Geometry: final body of the model. Coordinates: model frame, mm. A direction names the side the tool comes from. Give positions to 0.01 mm unless a question says otherwise; leave off trailing zeros. Loops run counter-clockwise (first coordinate to the right, second up) from the corner with the lowest first, then second, coordinate; pieces in that order, holes last. Notation, with made-up numbers: (79, -14) -> (87, -14) arc R20 ccw to (87, -6) -> close; hole circle Ø8 at (75.5, -1.75). An arc over 180 degrees is marked (long way). Answer in a Markdown table with one row per item. Add a question column.
1) Line query: line 1 (Y direction, x = -24, z = -18.75); line 2 (Z direction, x = -10, y = 42); line 3 (Z direction, x = 27.5, y = 4). Output: solid intervals per line, ascending. Write a range as from..to.
2) Draft query along Z for faces 6 (the flat face through (-10, 25, -22)), 7 (the flat face through (-22.7, 29.7, -10)), 8 (the flat face through (0, 29, -16)), 9 (the flat face through (-23.3, 29.7, 10)). Return one class per face: +Z half, -Z half, draft (parallel to the pull), parting line (faces both ways), or undercut.
3) Section query D-D (x = -24). Return the cut outline in (y, z), plus the area to 3 significant figures.
4) Access query for faces 1 (the flat face through (36, 8, 8)), 2 (the flat face through (12, 0, 0)), 3 (the flat face through (12, 16, 0)), 4 (the cylindrical face through (-19.386, 31.128, 16.084)), 5 (the flat face through (0, 29, 16)). Directions: +Z, -Z, +X, -X, +Y, -Y. A direction counts if a zero-diameter tool reaches every point of the face in a straight line with its end or side. Return the directions, or none.
5) Section query B-B (y = 7.5). Return the cut outline in (x, z).
6) Section query A-A (x = 46). Return the cut outline in (y, z), plus the area to 3 significant figures.
7) First-contact query: P1, Ø22, axis at x = 26.5, z = -7.5, coming from the +Y side; P2, Ø3.5, axis at y = 27.5, z = -16.5, coming from the +X side; P3, Ø3, axis at x = -21.5, z = 15.5, coming from the +Y side. Flat tips, straight axial feed; report the tip coordinate or a pass-through.
8) Section query C-C (z = 0). Return the cut outline in (x, y), plus the area to 3 significant figures.
```python
from build123d import *

# Parameters (mm, degrees)
BOSS_EXTRUDE1_DEPTH = 16
CUT_EXTRUDE2_DEPTH  = 16
SKETCH5_R           = 10
BOSS_EXTRUDE3_DEPTH = 12
SKETCH7_R           = 10
BOSS_EXTRUDE4_DEPTH = 12


with BuildPart() as part:
    # Sketch2 → Boss-Extrude1 (new body)
    with BuildSketch(Plane(origin=(0, 0, 0), x_dir=(1, 0, 0), z_dir=(0, 1, 0))):
        with BuildLine():
            Line((-48, 22), (48, 22))
            ThreePointArc((48, 22), (70, 0), (48, -22))
            Line((48, -22), (-48, -22))
            Line((-48, -22), (-48, 22))
        make_face()
    extrude(amount=BOSS_EXTRUDE1_DEPTH)

    # Sketch3 → Cut-Extrude2 (cut)
    with BuildSketch(Plane(origin=(0, 16, 0), x_dir=(1, 0, 0), z_dir=(0, 1, 0))):
        with BuildLine():
            Line((48, -8), (24, -8))
            ThreePointArc((24, -8), (16, 0), (24, 8))
            Line((24, 8), (48, 8))
            ThreePointArc((48, 8), (56, 0), (48, -8))
        make_face()
    extrude(amount=-CUT_EXTRUDE2_DEPTH, mode=Mode.SUBTRACT)

    # Sketch5 → Boss-Extrude3 (add)
    with BuildSketch(Plane.XY.offset(22)):
        with BuildLine():
            Line((-48, 40), (-48, 16))
            Line((-48, 16), (2, 16))
            ThreePointArc((2, 16), (0.585786438, 16.585786438), (0, 18))
            Line((0, 18), (0, 40))
            ThreePointArc((0, 40), (-24, 64), (-48, 40))
        make_face()
        with Locations((-24, 40)):
            Circle(SKETCH5_R, mode=Mode.SUBTRACT)
    extrude(amount=-BOSS_EXTRUDE3_DEPTH)

    # Sketch7 → Boss-Extrude4 (add)
    with BuildSketch(Plane(origin=(0, 0, -22), x_dir=(-1, 0, 0), z_dir=(0, 0, -1))):
        with BuildLine():
            Line((-2, 16), (48, 16))
            Line((48, 16), (48, 40))
            ThreePointArc((48, 40), (24, 64), (0, 40))
            Line((0, 40), (0, 18))
            ThreePointArc((0, 18), (-0.585786438, 16.585786438), (-2, 16))
        make_face()
        with Locations((24, 40)):
            Circle(SKETCH7_R, mode=Mode.SUBTRACT)
    extrude(amount=-BOSS_EXTRUDE4_DEPTH)


solid = part.part
```
Evaluation:
| question | item | result |
|---|---|---|
| 1 | line 1 | 0..30, 50..64 |
| 1 | line 2 | -22..-10, 10..22 |
| 1 | line 3 | -22..-8, 8..22 |
| 2 | face 6 | -Z half |
| 2 | face 7 | undercut |
| 2 | face 8 | draft |
| 2 | face 9 | undercut |
| 3 | outline | (0, -22) -> (30, -22) -> (30, -10) -> (16, -10) -> (16, 10) -> (30, 10) -> (30, 22) -> (0, 22) -> close; (50, -22) -> (64, -22) -> (64, -10) -> (50, -10) -> close; (50, 10) -> (64, 10) -> (64, 22) -> (50, 22) -> close |
| 3 | area | 1,380 mm² |
| 4 | face 1 | +Y, -Y |
| 4 | face 2 | +Z, -Z, +X, -X, -Y |
| 4 | face 3 | +X, +Y |
| 4 | face 4 | +Z, -Z |
| 4 | face 5 | +Z, -Z, +X, +Y |
| 5 | outline | (-48, -22) -> (48, -22) arc R22 ccw to (48, 22) -> (-48, 22) -> close; hole (24, -8) -> (48, -8) arc R8 ccw to (48, 8) -> (24, 8) arc R8 ccw to start |
| 6 | outline | (0, -22) -> (16, -22) -> (16, -8) -> (0, -8) -> close; (0, 8) -> (16, 8) -> (16, 22) -> (0, 22) -> close |
| 6 | area | 448 mm² |
| 7 | P1 | y = 16 |
| 7 | P2 | x = 0 |
| 7 | P3 | y = 63.98 |
| 8 | outline | (-48, 0) -> (16, 0) -> (16, 16) -> (-48, 16) -> close; (56, 0) -> (70, 0) -> (70, 16) -> (56, 16) -> close |
| 8 | area | 1,250 mm² |
